Could you check a few things on this model? Use its own coordinates, in mm. Coordinates: 2 decimals unless noted, no trailing zeros. Order: outer loops, then holes, each group sorted by start corner. A loop starts at its lowest first (then second) coordinate and runs counter-clockwise, first axis right, second up. Notation, with made-up numbers: (-23.75, -9.75) - (35.25, -9.75) arc R16 cw to (35.25, -5.75) - close; hole circle Ø7 at (71, 9). An arc over 180 degrees is marked (long way). One line per item, written item: value. Start each with the question number.
from build123d import *

# Parameters (mm, degrees)
EXTRUDE_1_DEPTH        = 400
SKETCH_2_R             = 3
SKETCH_2_R_2           = 1.75
CUT_EXTRUDE_1_DEPTH    = 4.5
SKETCH_2_2_R           = 1.75
CUT_EXTRUDE_2_DEPTH    = 9
PATTERN_LINEAR_1_COUNT = 16
PATTERN_LINEAR_1_PITCH = 25


with BuildPart() as part:
    # Эскиз1 → Бобышка-Вытянуть1 (new body)
    with BuildSketch(Plane.XY):
        with BuildLine():
            Line((-6, 3.7), (-5.7, 4))
            Line((-5.7, 4), (5.7, 4))
            Line((5.7, 4), (6, 3.7))
            Line((6, 3.7), (6, 2.451013544))
            ThreePointArc((6, 2.451013544), (5.597935912, 2.202976267), (5.354599002, 1.798050138))
            Line((5.354599002, 1.798050138), (4.643514056, 1.798050138))
            Line((4.643514056, 1.798050138), (4.643514056, 1.201949862))
            Line((4.643514056, 1.201949862), (5.354599002, 1.201949862))
            ThreePointArc((5.354599002, 1.201949862), (5.597935912, 0.797023733), (6, 0.548986456))
            Line((6, 0.548986456), (6, -3.7))
            Line((6, -3.7), (5.7, -4))
            Line((5.7, -4), (-5.7, -4))
            Line((-5.7, -4), (-6, -3.7))
            Line((-6, -3.7), (-6, 0.548986456))
            ThreePointArc((-6, 0.548986456), (-5.597935912, 0.797023733), (-5.354599002, 1.201949862))
            Line((-5.354599002, 1.201949862), (-4.643514056, 1.201949862))
            Line((-4.643514056, 1.201949862), (-4.643514056, 1.798050138))
            Line((-4.643514056, 1.798050138), (-5.354599002, 1.798050138))
            ThreePointArc((-5.354599002, 1.798050138), (-5.597935912, 2.202976267), (-6, 2.451013544))
            Line((-6, 2.451013544), (-6, 3.7))
        make_face()
    extrude(amount=EXTRUDE_1_DEPTH)

    # Эскиз2 → Вырез-Вытянуть1 (cut)
    with BuildSketch(Plane(origin=(0, 4, 0), x_dir=(1, 0, 0), z_dir=(0, 1, 0))):
        with Locations((0, -12)):
            Circle(SKETCH_2_R)
        with Locations((0, -12)):
            Circle(SKETCH_2_R_2, mode=Mode.SUBTRACT)
    cut_extrude_1 = extrude(amount=-CUT_EXTRUDE_1_DEPTH, mode=Mode.SUBTRACT)

    # Эскиз2<2> → Вырез-Вытянуть2 (cut, through all)
    with BuildSketch(Plane(origin=(0, 4, 0), x_dir=(1, 0, 0), z_dir=(0, 1, 0))):
        with Locations((0, -12)):
            Circle(SKETCH_2_2_R)
    cut_extrude_2 = extrude(amount=-CUT_EXTRUDE_2_DEPTH, mode=Mode.SUBTRACT)

    # Линейный массив1: Вырез-Вытянуть1, Вырез-Вытянуть2 ×16
    with Locations(*[(0, 0, i * PATTERN_LINEAR_1_PITCH) for i in range(1, PATTERN_LINEAR_1_COUNT)]):
        add(cut_extrude_1, mode=Mode.SUBTRACT)
        add(cut_extrude_2, mode=Mode.SUBTRACT)


solid = part.part
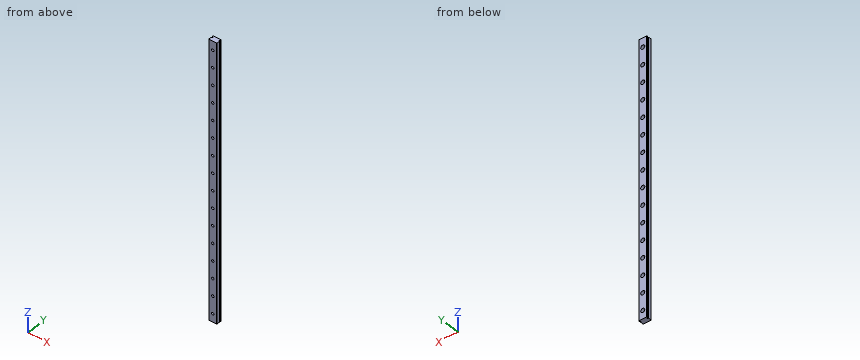
Q1. I'm going to push flat-ended pins straight in: pin 1 (5.5 mm diameter, centred on x = 0, z = 112, fed in from +Y); pin 2 (1.5 mm diameter, centred on y = 1.5, z = 155, fed in from +X); pin 3 (0.5 mm diameter, centred on y = 1.5, z = 152.5, fed in from -X); pin 4 (3 mm diameter, centred on x = 0, z = 237, fed in from -Y). Where does each tip first touch, or does it pass through?
Q2. If I drill on L1, parallel to X at y = -1.75, z = 262; L2, parallel to X at y = 1.25, z = 311.5; L3, parallel to Y at x = 5.25, z = 88, over which ranges is the centre line in solid material (lowest first)?
Q3. I want a section at B-B on y = -2. State how many separate pieces and enclosed holes the cut face has, then the cut area to 3 significant figures.
Q4. I want a section at A-A on z = 278.5. Please give me the cut outline in (x, y), then the cut area to 3 significant figures.
Values follow:
1. pin 1: stops at y = -0.5
1. pin 2: stops at x = 5.65
1. pin 3: stops at x = -4.64
1. pin 4: passes through
2. L1: x = -6 to -1.75, 1.75 to 6
2. L2: x = -4.64 to -2.96, 2.96 to 4.64
2. L3: y = -4 to 1.2, 1.8 to 4
3. separate pieces: 1
3. enclosed holes: 16
3. area: 4,650 mm^2
4. outline: (-6, -3.7) - (-5.7, -4) - (5.7, -4) - (6, -3.7) - (6, 0.55) arc R1 cw to (5.35, 1.2) - (4.64, 1.2) - (4.64, 1.8) - (5.35, 1.8) arc R1 cw to (6, 2.45) - (6, 3.7) - (5.7, 4) - (-5.7, 4) - (-6, 3.7) - (-6, 2.45) arc R1 cw to (-5.35, 1.8) - (-4.64, 1.8) - (-4.64, 1.2) - (-5.35, 1.2) arc R1 cw to (-6, 0.55) - close
4. area: 93.1 mm^2
